Check sheet for the modelled part. Datum: model origin and axes. Units: mm. A direction names the side the tool comes from. Give positions to 0.01 mm unless a question says otherwise; leave off trailing zeros. Write each loop counter-clockwise with the first axis right and the second up, starting at its lowest first coordinate (ties: lowest second). Pieces come first, ordered by that corner, then holes. Notation, with made-up numbers: M 65,19 L 75,19 A21 ccw 75,35 Z; hole C 61.25,57.5 d4. An arc over 180 degrees is marked long. Write item = value, one per line. Start each with the question number.
1) Access from +Z, -Z, +X, -X, +Y, -Y to the whole of each face (thin tool, end or side, straight path). Record for faces 1 (the cylindrical face through (25.855, 5.716, 21.432)), 2 (the cylindrical face through (-6.58, 11.63, 15.7)), 3 (the flat face through (-20.15, 0, 10)).
2) Cross-section at C-C, the plane z = 14.95. Give the number of separate pieces and of enclosed holes in the cut face, plus the area to 3 significant figures.
3) Scan lines: line 1 along Y through (x, z) = (-2.5, 19.75); line 2 along Y through (x, z) = (24, 8.25); line 3 along Y through (x, z) = (-23.5, 12). Record each from-to range of solid material in increasing order. Write a range as [from, to].
4) Cross-section at A-A, the plane y = -5.1. Record the cut outline in (x, z), plus the area to 3 significant figures.
5) Cross-section at D-D, the plane x = 3. Record the cut outline in (y, z).
6) Mould release check, pull along X, two halves, no side actions. Record for faces 4 (the cylindrical face through (-18.58, 11.63, 15.7)), 5 (the flat face through (25.5, 11.4, 10)), 6 (the flat face through (0, 13.15, 10)): released by +X, released by -X, zero draft, split by the parting line, or undercut.
7) Cross-section at B-B, the plane x = -6. Record the cut outline in (y, z), plus the area to 3 significant figures.
8) Go/stop test with a flat-tipped pin: pin 1 (3 mm diameter, centred on x = 23.9, y = 5.1, fed in from +Z). Record where the tip stops, or that it passes through.
```python
from build123d import *

# Parameters (mm, degrees)
SKETCH_1_W          = 54.5
SKETCH_1_H          = 26.3
SKETCH_1_R          = 0.95
SKETCH_1_W_2        = 40.3
SKETCH_1_H_2        = 20.3
EXTRUDE_1_DEPTH     = 20.2
SKETCH_2_R          = 2.05
SKETCH_2_R_2        = 0.95
EXTRUDE_2_DEPTH     = 2.5
CHAMFER_1_SIZE      = 3.5
SKETCH_3_R          = 0.95
CUT_EXTRUDE_1_DEPTH = 45.15362386
SKETCH_4_R          = 0.95
CUT_EXTRUDE_2_DEPTH = 45.15362386
SKETCH_5_W          = 7.1
SKETCH_5_H          = 6.1
CUT_EXTRUDE_3_DEPTH = 37.380283121


with BuildPart() as part:
    # 스케치1 → 보스-돌출1 (new body)
    with BuildSketch(Plane.XY):
        Rectangle(SKETCH_1_W, SKETCH_1_H)
        with Locations((-23.9, 5.1)):
            Circle(SKETCH_1_R, mode=Mode.SUBTRACT)
        with Locations((23.9, 5.1)):
            Circle(SKETCH_1_R, mode=Mode.SUBTRACT)
        with Locations((23.9, -5.1)):
            Circle(SKETCH_1_R, mode=Mode.SUBTRACT)
        with Locations((-23.9, -5.1)):
            Circle(SKETCH_1_R, mode=Mode.SUBTRACT)
        Rectangle(SKETCH_1_W_2, SKETCH_1_H_2, mode=Mode.SUBTRACT)
    extrude(amount=EXTRUDE_1_DEPTH)

    # 스케치2 → 보스-돌출2 (add)
    # profile 1 of 4: a face of its own
    with BuildSketch(Plane.XY.offset(20.2)):
        with Locations((-23.9, 5.1)):
            Circle(SKETCH_2_R)
        with Locations((-23.9, 5.1)):
            Circle(SKETCH_2_R_2, mode=Mode.SUBTRACT)
    # profile 2 of 4: a face of its own
    with BuildSketch(Plane.XY.offset(20.2)):
        with Locations((-23.9, -5.1)):
            Circle(SKETCH_2_R)
        with Locations((-23.9, -5.1)):
            Circle(SKETCH_2_R_2, mode=Mode.SUBTRACT)
    # profile 3 of 4: a face of its own
    with BuildSketch(Plane.XY.offset(20.2)):
        with Locations((23.9, 5.1)):
            Circle(SKETCH_2_R)
        with Locations((23.9, 5.1)):
            Circle(SKETCH_2_R_2, mode=Mode.SUBTRACT)
    # profile 4 of 4: a face of its own
    with BuildSketch(Plane.XY.offset(20.2)):
        with Locations((23.9, -5.1)):
            Circle(SKETCH_2_R)
        with Locations((23.9, -5.1)):
            Circle(SKETCH_2_R_2, mode=Mode.SUBTRACT)
    extrude(amount=EXTRUDE_2_DEPTH)

    # 모따기1
    chamfer_1_edges = [part.edges().sort_by_distance(p)[0] for p in [
        (27.25, 13.15, 10.1),
        (27.25, -13.15, 10.1),
        (-27.25, -13.15, 10.1),
        (-27.25, 13.15, 10.1),
    ]]
    chamfer(chamfer_1_edges, length=CHAMFER_1_SIZE)

    # 스케치3 → 컷-돌출1 (cut, through all)
    with BuildSketch(Plane.XZ.offset(13.15)):
        with Locations(Location((-6, 14.95, 0), (0, 0, 270))):
            Circle(SKETCH_3_R)
        with Locations(Location((6, 14.95, 0), (0, 0, 270))):
            Circle(SKETCH_3_R)
        with Locations(Location((-18, 14.95, 0), (0, 0, 270))):
            Circle(SKETCH_3_R)
        with Locations(Location((18, 14.95, 0), (0, 0, 270))):
            Circle(SKETCH_3_R)
    extrude(amount=-CUT_EXTRUDE_1_DEPTH, mode=Mode.SUBTRACT)

    # 스케치4 → 컷-돌출2 (cut, through all)
    with BuildSketch(Plane.XZ.offset(13.15)):
        with Locations(Location((-6, 4.75, 0), (0, 0, 270))):
            Circle(SKETCH_4_R)
        with Locations(Location((6, 4.75, 0), (0, 0, 270))):
            Circle(SKETCH_4_R)
        with Locations(Location((-18, 4.75, 0), (0, 0, 270))):
            Circle(SKETCH_4_R)
        with Locations(Location((18, 4.75, 0), (0, 0, 270))):
            Circle(SKETCH_4_R)
    extrude(amount=-CUT_EXTRUDE_2_DEPTH, mode=Mode.SUBTRACT)

    # 스케치5 → 컷-돌출3 (cut, through all)
    with BuildSketch(Plane.XY.offset(20.2)):
        with Locations((23.7, 0)):
            Rectangle(SKETCH_5_W, SKETCH_5_H)
    extrude(amount=-CUT_EXTRUDE_3_DEPTH, mode=Mode.SUBTRACT)


solid = part.part
```
Reply:
q1.face_1 = +Z
q1.face_2 = +Y, -Y
q1.face_3 = +Z, -Z
q2.separate_pieces = 9
q2.enclosed_holes = 4
q2.area = 491 mm2
q3.line_1 = [-13.15, -10.15], [10.15, 13.15]
q3.line_2 = [-12.9, -6.04], [-4.16, -3.05], [3.05, 4.16], [6.04, 12.9]
q3.line_3 = [-13.15, -5.96], [-4.24, 4.24], [5.96, 13.15]
q4.outline = M -27.25,0 L -24.85,0 L -24.85,22.7 L -25.95,22.7 L -25.95,20.2 L -27.25,20.2 Z; M -22.95,0 L -20.15,0 L -20.15,20.2 L -21.85,20.2 L -21.85,22.7 L -22.95,22.7 Z; M 20.15,0 L 22.95,0 L 22.95,22.7 L 21.85,22.7 L 21.85,20.2 L 20.15,20.2 Z; M 24.85,0 L 27.25,0 L 27.25,20.2 L 25.95,20.2 L 25.95,22.7 L 24.85,22.7 Z
q4.area = 221 mm2
q5.outline = M -13.15,0 L -10.15,0 L -10.15,20.2 L -13.15,20.2 Z; M 10.15,0 L 13.15,0 L 13.15,20.2 L 10.15,20.2 Z
q6.face_4 = undercut
q6.face_5 = released by +X
q6.face_6 = zero draft
q7.outline = M -13.15,0 L -10.15,0 L -10.15,3.8 L -13.15,3.8 Z; M -13.15,5.7 L -10.15,5.7 L -10.15,14 L -13.15,14 Z; M -13.15,15.9 L -10.15,15.9 L -10.15,20.2 L -13.15,20.2 Z; M 10.15,0 L 13.15,0 L 13.15,3.8 L 10.15,3.8 Z; M 10.15,5.7 L 13.15,5.7 L 13.15,14 L 10.15,14 Z; M 10.15,15.9 L 13.15,15.9 L 13.15,20.2 L 10.15,20.2 Z
q7.area = 98.4 mm2
q8.pin_1 = 22.7
